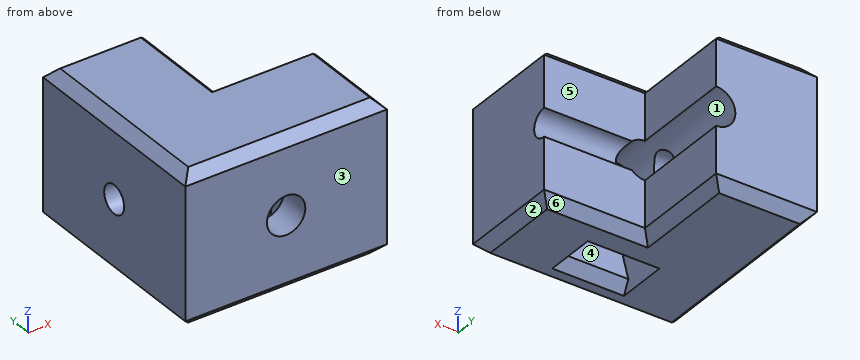
from build123d import *

# Parameters (mm, degrees)
BOSS_EXTRUDE2_DEPTH     = 15
SKETCH3_R               = 1.4
CUT_EXTRUDE1_DEPTH      = 33.015621187
CUT_EXTRUDE2_DEPTH      = 31.232432916
CUT_EXTRUDE2_DEPTH_BACK = 31.232432916
SKETCH4_R               = 1.9
CUT_EXTRUDE3_DEPTH      = 3
CHAMFER1_SIZE           = 1
CHAMFER2_SIZE           = 1
CHAMFER5_SIZE           = 1


with BuildPart() as part:
    # Sketch2 → Boss-Extrude2 (new body)
    with BuildSketch(Plane.XY):
        Polygon((0, 20), (0, 0), (20, 0), (20, 10), (10, 10), (10, 20), align=None)
    extrude(amount=BOSS_EXTRUDE2_DEPTH)

    # Sketch3 → Cut-Extrude1 (cut, through all)
    with BuildSketch(Plane.ZY):
        with Locations((7.5, 10)):
            Circle(SKETCH3_R)
    extrude(amount=-CUT_EXTRUDE1_DEPTH, mode=Mode.SUBTRACT)

    # Sketch4 → Cut-Extrude2 (cut, two sides: drawn at the far end of the back side and taken through both)
    with BuildSketch(Plane(origin=(0, 3, 0), x_dir=(-1, 0, 0), z_dir=(0, -1, 0)).offset(-CUT_EXTRUDE2_DEPTH_BACK)):
        with Locations(Location((-10, -7.5, 0), (0, 0, 90))):
            Circle(SKETCH4_R)
    extrude(amount=CUT_EXTRUDE2_DEPTH + CUT_EXTRUDE2_DEPTH_BACK, mode=Mode.SUBTRACT)

    # Sketch5 → Cut-Extrude3 (cut)
    with BuildSketch(Plane(origin=(0, 3, 0), x_dir=(-1, 0, 0), z_dir=(0, -1, 0))):
        Polygon((-12.75, -3), (-13.553847577, 0), (-6.446152423, 0), (-7.25, -3), (-7.25, -12), (-12.75, -12), align=None)
    extrude(amount=-CUT_EXTRUDE3_DEPTH, mode=Mode.SUBTRACT)

    # Chamfer1
    chamfer1_edges = [part.edges().sort_by_distance(p)[0] for p in [
        (10, 3, 0),
        (10, 6, 0),
    ]]
    chamfer(chamfer1_edges, length=CHAMFER1_SIZE)

    # Chamfer2
    chamfer2_edges = [part.edges().sort_by_distance(p)[0] for p in [
        (10, 0, 15),
        (20, 5, 15),
        (15, 10, 15),
        (10, 15, 15),
        (5, 20, 15),
        (0, 10, 15),
    ]]
    chamfer(chamfer2_edges, length=CHAMFER2_SIZE)

    # Chamfer5
    chamfer5_edges = [part.edges().sort_by_distance(p)[0] for p in [
        (10, 15, 0),
        (15, 10, 0),
        (20, 5, 0),
        (10, 0, 0),
        (0, 10, 0),
        (5, 20, 0),
    ]]
    chamfer(chamfer5_edges, length=CHAMFER5_SIZE)


solid = part.part
Source: CAD feature listing. Evaluate the final solid. Frame: model axes, mm. Face numbers are marked on the shaded views. A direction names the side the tool comes from. Round coordinates to 2 decimals unless told otherwise and drop trailing zeros. Loops run counter-clockwise (first coordinate to the right, second up) from the corner with the lowest first, then second, coordinate; pieces in that order, holes last. Notation, with made-up numbers: (74, 10) - (87, 10) arc R20 cw to (87, 21) - close; hole circle Ø2 at (16, 48). An arc over 180 degrees is marked (long way). Write item = value, one per line. Start each with the question number.
(1) Set-up query: the marked faces 4, 5 and 6. Return all of +Z, -Z, +X, -X, +Y, -Y with unobstructed straight access to the full face (end or side cutting, diameter ignored); none if empty.
(2) Pull-direction query (Z, two-part tool) for the marked faces 1, 2 and 3; classes: +Z half, -Z half, draft (parallel to the pull), parting line (faces both ways), or undercut.
(3) Section query D-D, the plane x = 17. Output: boundary loops of the cut face in (y, z).
(4) Ray query, line 1 along Z through (x, y) = (2.75, 10); line 2 along Z through (x, y) = (10, 1.9); line 3 along Y through (x, z) = (12.75, 2). Return the intervals inside material, ascending. Write a range as from..to.
(5) Section query B-B, the plane z = 7.5. Output: boundary loops of the cut face in (x, y), plus the area to 3 significant figures.
(6) Section query A-A, the plane z = 10.75. Output: boundary loops of the cut face in (x, y).
(7) Pin query (flat end, axial travel): pin 1 (2.5 mm diameter, centred on y = 15, z = 12.5, fed in from +X); pin 2 (8 mm diameter, centred on x = 13, y = 12.5, fed in from +Z); pin 3 (2.5 mm diameter, centred on x = 16.5, z = 11.5, fed in from +Y); pin 4 (3.5 mm diameter, centred on x = 10.5, y = 4, fed in from -Z). Return the tip coordinate at first contact, or that it passes through.
(8) Section query C-C, the plane y = 11.75. Output: boundary loops of the cut face in (x, z).
Conclusion:
q1.face_4 = -Z
q1.face_5 = +Z, -Z, +X, +Y
q1.face_6 = -Z, +X, +Y
q2.face_1 = undercut
q2.face_2 = -Z half
q2.face_3 = draft
q3.outline = (0, 1) - (1, 0) - (9, 0) - (10, 1) - (10, 6.1) arc R1.4 cw to (10, 8.9) - (10, 14) - (9, 15) - (1, 15) - (0, 14) - close
q4.line_1 = 0..6.1, 8.9..15
q4.line_2 = 0..5.6, 9.4..15
q4.line_3 = 0..3, 6..10
q5.outline = (0, 0) - (8.1, 0) - (8.1, 3) - (7.25, 3) - (7.25, 6) - (8.1, 6) - (8.1, 8.6) - (0, 8.6) - close; (0, 11.4) - (8.1, 11.4) - (8.1, 20) - (0, 20) - close; (11.9, 0) - (20, 0) - (20, 8.6) - (11.9, 8.6) - (11.9, 6) - (12.75, 6) - (12.75, 3) - (11.9, 3) - close
q5.area = 204 mm2
q6.outline = (0, 0) - (20, 0) - (20, 10) - (10, 10) - (10, 20) - (0, 20) - close; hole (7.25, 3) - (12.75, 3) - (12.75, 6) - (7.25, 6) - close
q7.pin_1 = 10
q7.pin_2 = 15
q7.pin_3 = 10
q7.pin_4 = 0.25
q8.outline = (0, 1) - (1, 0) - (9, 0) - (10, 1) - (10, 5.6) arc R1.9 cw to (10, 9.4) - (10, 14) - (9, 15) - (1, 15) - (0, 14) - close
